Could you check a few things on this model? Use its own coordinates, in mm. Face numbers are marked on the shaded views. A direction names the side the tool comes from. Round coordinates to 2 decimals unless told otherwise and drop trailing zeros. Loops run counter-clockwise (first coordinate to the right, second up) from the corner with the lowest first, then second, coordinate; pieces in that order, holes last. Notation, with made-up numbers: (-24, -13.75) -> (-16, -13.75) arc R24 cw to (-16, -3.75) -> close; hole circle Ø4 at (49, -34). An arc over 180 degrees is marked (long way). Write each question's results on one line, items separated by ' | '. Start each with the question number.
1) We'd pull the mould along X, two halves only. Please class the marked faces 1, 2, 3 and 4: pulls with the +X half, pulls with the -X half, needs draft (parallel to the pull), parting line crosses it, or undercut.
2) Which directions (+Z, -Z, +X, -X, +Y, -Y) give clear straight access to the entire face, cutting with the end or side of a thin tool? Please do the marked faces 5, 6 and 7.
3) Imagine slicing it at C-C, the plane z = 43. List the corners of the cut face in (x, y) for me.
4) Imagine slicing it at A-A, the plane z = 6.5. List the corners of the cut face in (x, y) for me.
5) Imagine slicing it at D-D, the plane x = 83. List the corners of the cut face in (y, z) for me, plus the area to 3 significant figures.
6) If I drill on probe 1 along X at (y, z) = (-48.5, 32); probe 2 along X at (y, z) = (-107, 36.5); probe 3 along Z at (x, y) = (-97, -13.5), over which ranges is the centre line in solid material (lowest first)?
7) For P1, Ø3, axis at y = -99.5, z = 21.5, coming from the -X side; P2, Ø11.5, axis at x = 122, z = 37, coming from the +Y side; P3, Ø16, axis at y = -79.5, z = 40.5, coming from the -X side; P4, Ø12, axis at x = 27.5, z = 7.5, coming from the +Y side, each with a flat end and sliding along its axis, tell me the tip position at first contact or that it passes through.
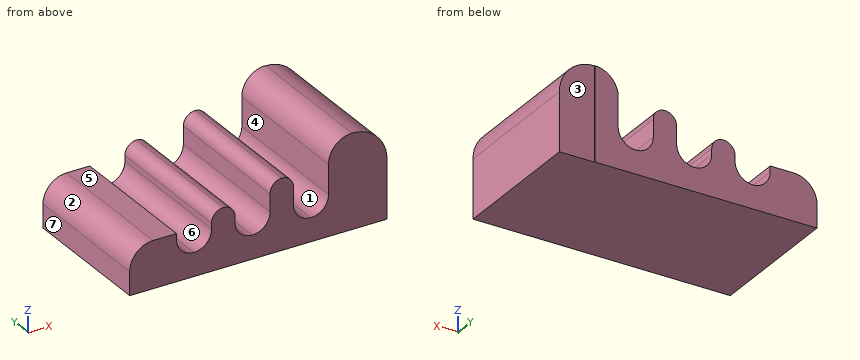
from build123d import *

# Parameters (mm, degrees)
F0_W      = 12.7
F0_H      = 25.4
F0_W_2    = 25.4
F1_DEPTH  = 152.4
F2_W      = 152.4
F2_H      = 25.4
F3_DEPTH  = 38.1
F4_R      = 25.4
F6_DEPTH  = 151.892
F7_R      = 19.05
F8_R      = 19.04999
F9_R      = 19.04999
F10_R     = 12.69999
F11_R     = 25.39999
F12_ANGLE = 90


# Not quite as in the source:
# - a fillet or chamfer is up to 0.001 mm smaller than in the source, because OpenCascade refuses the exact size


with BuildPart() as f1:
    # F0 (on Front) → F1 (new body)
    with BuildSketch(Plane.XZ):
        Polygon((-147.5200289965, 215.9), (-172.9200289965, 215.9), (-249.1200289965, 215.9), (-249.1200289965, 190.5), (-172.9200289965, 190.5), (-172.9200289965, 152.4), (-223.7200289965, 152.4), (-223.7200289965, 127), (-172.9200289965, 127), (-172.9200289965, 88.9), (-211.0200289965, 88.9), (-211.0200289965, 63.5), (-172.9200289965, 63.5), (-172.9200289965, 25.4), (-172.9200289965, 0), (-160.2200289965, 0), (-147.5200289965, 0), (-147.5200289965, 63.5), (-147.5200289965, 88.9), (-147.5200289965, 127), (-147.5200289965, 152.4), (-147.5200289965, 190.5), align=None)
        with Locations((-153.8700289965, -12.7)):
            Rectangle(F0_W, F0_H)
        with Locations((-185.6200289965, 12.7)):
            Rectangle(F0_W_2, F0_H)
    extrude(amount=F1_DEPTH)

    # F2 (on face) → F3 (join)
    with BuildSketch(Plane(origin=(-160.2200289965, 0, 0), x_dir=(0, -1, 0), z_dir=(-1, 0, 0))):
        with Locations((76.2, -12.7)):
            Rectangle(F2_W, F2_H)
    extrude(amount=F3_DEPTH)

    # F4
    f4_edges = [f1.edges().sort_by_distance(p)[0] for p in [
        (-198.320029, -76.2, -25.4),
    ]]
    fillet(f4_edges, radius=F4_R)

    # F5 (on face) → F6 (join)
    with BuildSketch(Plane.XZ.offset(152.4)):
        with BuildLine():
            ThreePointArc((-211.0200289965, 254), (-237.9607973597, 242.8407683632), (-249.1200289965, 215.9))
            Line((-249.1200289965, 215.9), (-147.5200289965, 215.9))
            Line((-147.5200289965, 215.9), (-147.5200289965, 254))
            Line((-147.5200289965, 254), (-211.0200289965, 254))
        make_face()
    extrude(amount=-F6_DEPTH)

    # F7
    f7_edges = [f1.edges().sort_by_distance(p)[0] for p in [
        (-172.920029, -76.2, 88.9),
    ]]
    fillet(f7_edges, radius=F7_R)

    # F8 (radius 19.05 in the source; OpenCascade refuses exactly that, so slightly less here)
    f8_edges = [f1.edges().sort_by_distance(p)[0] for p in [
        (-172.920029, -76.2, 190.5),
        (-172.920029, -76.2, 127),
    ]]
    fillet(f8_edges, radius=F8_R)

    # F9 (radius 19.05 in the source; OpenCascade refuses exactly that, so slightly less here)
    f9_edges = [f1.edges().sort_by_distance(p)[0] for p in [
        (-172.920029, -76.2, 152.4),
        (-172.920029, -76.2, 25.4),
        (-172.920029, -76.2, 63.5),
    ]]
    fillet(f9_edges, radius=F9_R)

    # F10 (radius 12.7 in the source; OpenCascade refuses exactly that, so slightly less here)
    f10_edges = [f1.edges().sort_by_distance(p)[0] for p in [
        (-223.720029, -76.2, 152.4),
        (-223.720029, -76.2, 127),
        (-211.020029, -76.2, 88.9),
        (-211.020029, -76.2, 63.5),
    ]]
    fillet(f10_edges, radius=F10_R)

    # F11 (radius 25.4 in the source; OpenCascade refuses exactly that, so slightly less here)
    f11_edges = [f1.edges().sort_by_distance(p)[0] for p in [
        (-249.120029, -76.2, 190.5),
    ]]
    fillet(f11_edges, radius=F11_R)


with BuildPart() as f1_1:
    # F12: moved
    add(f1.part.rotate(Axis((-147.5200289965, -76.2, -25.4), (0, 1, 0)), F12_ANGLE))


solid = f1_1.part
Checked values:
1) face 1: undercut | face 2: pulls with the -X half | face 3: needs draft | face 4: undercut
2) face 5: +Z, -X, +Y, -Y | face 6: +Z, +Y, -Y | face 7: +Z, -Z, -X, +Y, -Y
3) outline: (5.86, -152.4) -> (29.3, -152.4) -> (29.3, 0) -> (5.86, 0) -> close; (68.38, -152.4) -> (131.56, -152.4) -> (131.56, -0.51) -> (93.78, -0.51) -> (93.78, 0) -> (68.38, 0) -> close
4) outline: (-146.67, -152.4) -> (-92, -152.4) -> (-92, 0) -> (-146.67, 0) -> close; (-63.34, -152.4) -> (-28.5, -152.4) -> (-28.5, 0) -> (-63.34, 0) -> close; (0.16, -152.4) -> (35, -152.4) -> (35, 0) -> (0.16, 0) -> close; (63.66, -152.4) -> (131.88, -152.4) -> (131.88, -0.51) -> (93.78, -0.51) -> (93.78, 0) -> (63.66, 0) -> close
5) outline: (-152.4, -25.4) -> (0, -25.4) -> (0, 73.8) -> (-152.4, 73.8) -> close | area: 15,100 mm^2
6) probe 1: -56.77 to -35.07, 4.88 to 30.28, 68.38 to 131.88 | probe 2: -52.09 to -39.75, 4.88 to 30.28, 68.38 to 131.88 | probe 3: -25.4 to 25.4
7) P1: x = -137.78 | P2: y = -0.51 | P3: x = -56.45 | P4: y = 0
